Could you check a few things on this drawing? It's one solid part, dimensions in mm from its lowest x, y, z. A direction names the side the tool comes from. Coordinates: 2 decimals unless noted, no trailing zeros. Loops run counter-clockwise (first coordinate to the right, second up) from the corner with the lowest first, then second, coordinate; pieces in that order, holes last.
1) Thinking about a two-plate mould opening in Y: for the marked faces 3, 4 and 5, which applies, released by +Y, released by -Y, zero draft, split by the parting line, or undercut?
2) Imagine slicing it at C-C on x = 4. Give the number of separate pieces and of enclosed holes in the cut face, plus the area to 3 significant figures.
3) Will these pins go through, and if not, where does the flat tip stop? P1, Ø4.5, axis at x = 12, z = 13, coming from the +Y side; P2, Ø1, axis at x = 10.5, y = 15, coming from the +Z side; P3, Ø2.5, axis at x = 20, z = 5, coming from the +Y side.
4) If I drill on line 1 along Y through (x, z) = (20, 1.2); line 2 along X through (y, z) = (1.45, 5); line 3 along X through (y, z) = (1.5, 12), over which ranges is the centre line in solid material (lowest first)?
5) For the marked faces 1 and 2, which set-ups out of +Z, -Z, +X, -X, +Y, -Y let a thin tool reach every point of the face, with its end or its side?
6) Imagine slicing it at A-A on y = 6. Please give me the cut outline in (x, z), plus the area to 3 significant figures.
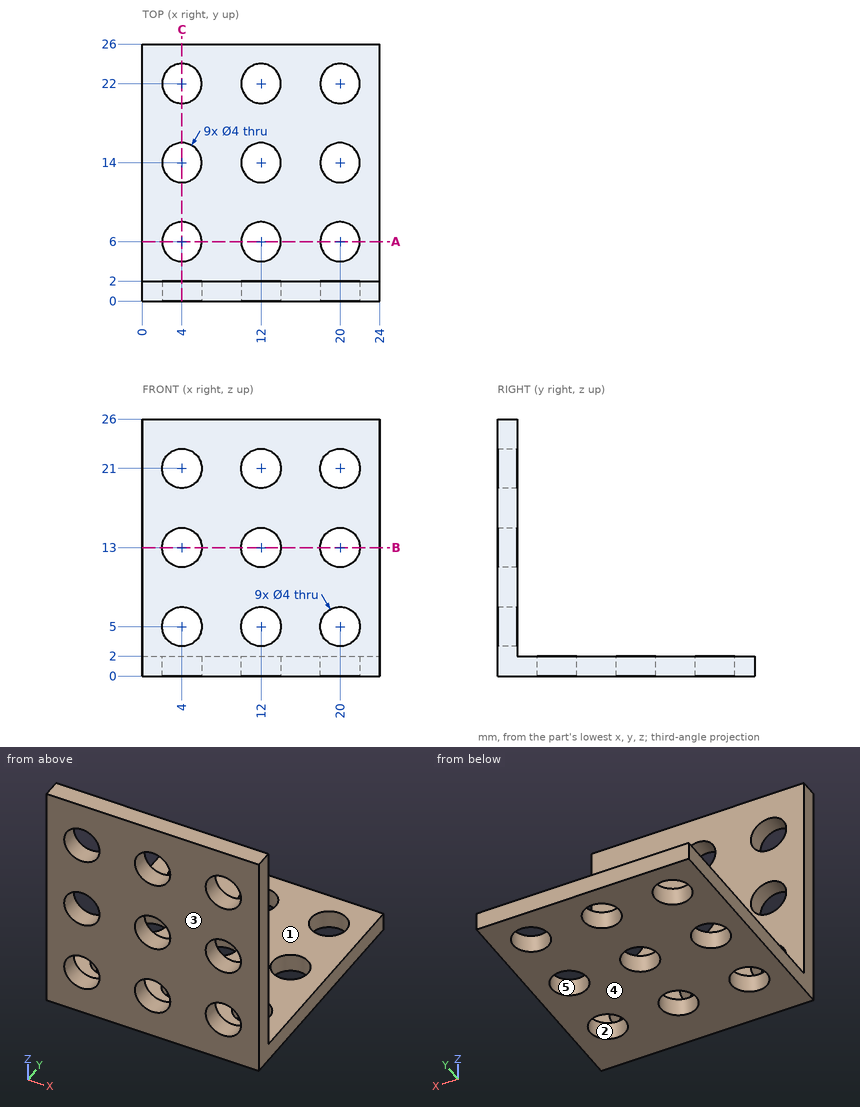
Filled in:
1. face 3: released by -Y
1. face 4: zero draft
1. face 5: undercut
2. separate pieces: 7
2. enclosed holes: 0
2. area: 52.0 mm2
3. P1: stops at y = 2
3. P2: stops at z = 2
3. P3: passes through
4. line 1: y = 0 to 4, 8 to 12, 16 to 20, 24 to 26
4. line 2: x = 0 to 2, 6 to 10, 14 to 18, 22 to 24
4. line 3: x = 0 to 2.27, 5.73 to 10.27, 13.73 to 18.27, 21.73 to 24
5. face 1: +Z, +X, -X, +Y
5. face 2: +Z, -Z
6. outline: (0, 0) - (2, 0) - (2, 2) - (0, 2) - close; (6, 0) - (10, 0) - (10, 2) - (6, 2) - close; (14, 0) - (18, 0) - (18, 2) - (14, 2) - close; (22, 0) - (24, 0) - (24, 2) - (22, 2) - close
6. area: 24.0 mm2
